```python
from build123d import *

# Parameters (mm, degrees)
F1_DEPTH = 13.2296
F2_R     = 2.93654


with BuildPart() as f1:
    # F0 (on Top) → F1 (new body)
    with BuildSketch(Plane.XY):
        Polygon((7.648975, 63.29149), (0, 63.29149), (-9.748682, 59.991933), (-10.348603, 54.892614), (-15.89787, 48.443481), (-20.847201, 42.594269), (-10.198623, 34.345381), (3.59951, 36.145136), (14.398068, 36.445096), (25.496572, 38.544811), (25.946513, 47.5436), (20.547241, 53.842753), (13.198227, 53.842753), (7.648975, 57.742231), align=None)
    extrude(amount=F1_DEPTH)

    # F2
    f2_edges = [f1.edges().sort_by_distance(p)[0] for p in [
        (-9.748682, 59.991933, 6.6148),
    ]]
    fillet(f2_edges, radius=F2_R)


solid = f1.part
```
For this review, take the finished solid that the model builds, in its own axes (mm). A direction names the side the tool comes from. Coordinates: 2 decimals unless noted, no trailing zeros. Loops run counter-clockwise (first coordinate to the right, second up) from the corner with the lowest first, then second, coordinate; pieces in that order, holes last. Notation, with made-up numbers: (53, 71) - (68, 71) arc R25 ccw to (68, 92) - close; hole circle Ø9 at (-0.75, 36). An arc over 180 degrees is marked (long way). Use one line per item in the form item = value. Start each with the question number.
1) For pin 1 (6 mm diameter, centred on y = 43.5, z = 2.5, fed in from -X); pin 2 (6 mm diameter, centred on x = 16, z = 4.5, fed in from -Y); pin 3 (6 mm diameter, centred on y = 47, z = 10, fed in from -X); pin 4 (3 mm diameter, centred on y = 60, z = 8.5, fed in from +X), all flat-tipped, find the tip position at first contact; note any pin that passes through.
2) Take a section at B-B (x = -13.5). State the section outline as (y, z) points, plus the area to 3 significant figures.
3) To check wall thickness, follow probe 1 along X at (y, z) = (52.25, 8.25); probe 2 along X at (y, z) = (55, 2.5); probe 3 along Y at (x, z) = (11, 2.5). State the ranges of each line that lie inside material, in increasing order. Write a range as from..to.
4) For faces 1 (the face through (4, 63.291, 7)), 2 (the face through (17, 53.843, 7)), list the 3-axis set-ups (+Z, -Z, +X, -X, +Y, -Y) from which the entire face can be reached by the end or side of a thin tool; tool diameter is ignored.
5) Take a section at C-C (y = 50). State the section outline as (x, z) points, plus the area to 3 significant figures.
6) Take a section at A-A (z = 11.25). State the section outline as (x, y) points, plus the area to 3 significant figures.
From the geometry:
q1.pin_1 = -20.85
q1.pin_2 = 36.41
q1.pin_3 = -19.66
q1.pin_4 = 7.65
q2.outline = (36.9, 0) - (51.23, 0) - (51.23, 13.23) - (36.9, 13.23) - close
q2.area = 190 mm2
q3.probe_1 = -12.62..21.91
q3.probe_2 = -10.34..11.55
q3.probe_3 = 36.35..55.39
q4.face_1 = +Z, -Z, +X, -X, +Y
q4.face_2 = +Z, -Z, +X, +Y
q5.outline = (-14.56, 0) - (23.84, 0) - (23.84, 13.23) - (-14.56, 13.23) - close
q5.area = 508 mm2
q6.outline = (-20.85, 42.59) - (-10.2, 34.35) - (3.6, 36.15) - (14.4, 36.45) - (25.5, 38.54) - (25.95, 47.54) - (20.55, 53.84) - (13.2, 53.84) - (7.65, 57.74) - (7.65, 63.29) - (0, 63.29) - (-7.99, 60.59) arc R2.94 ccw to (-9.97, 58.15) - (-10.35, 54.89) - (-15.9, 48.44) - close
q6.area = 887 mm2
